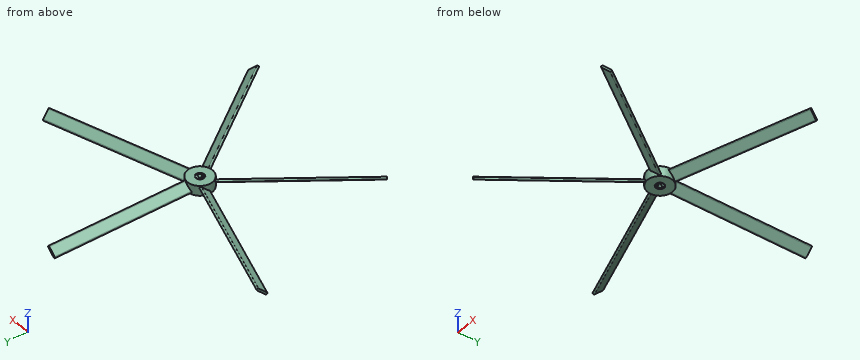
```python
from build123d import *

# Parameters (mm, degrees)
SKETCH1_R           = 7.5
SKETCH1_R_2         = 2.5
BOSS_EXTRUDE1_DEPTH = 6
BOSS_EXTRUDE2_DEPTH = 88.9
CIRPATTERN1_COUNT   = 5


with BuildPart() as part:
    # Sketch1 → Boss-Extrude1 (new body)
    with BuildSketch(Plane.XY):
        Circle(SKETCH1_R)
        Circle(SKETCH1_R_2, mode=Mode.SUBTRACT)
    extrude(amount=BOSS_EXTRUDE1_DEPTH)

    # Sketch3 → Boss-Extrude2 (add)
    with BuildSketch(Plane(origin=(0, 0, 0), x_dir=(1, 0, 0), z_dir=(0, 1, 0))):
        with BuildLine():
            Line((-2.427610564, -1.81062126), (1.710616437, -5.267397014))
            ThreePointArc((1.710616437, -5.267397014), (2.617021972, -5.186071015), (2.535695974, -4.27966548))
            Line((2.535695974, -4.27966548), (-1.602531027, -0.822889726))
            ThreePointArc((-1.602531027, -0.822889726), (-2.508936562, -0.904215725), (-2.427610564, -1.81062126))
        make_face()
    boss_extrude2 = extrude(amount=BOSS_EXTRUDE2_DEPTH)

    # CirPattern1: Boss-Extrude2 ×5 about axis
    cirpattern1_axis = Axis((0, 0, 0), (0, 0, 1))
    for i in range(1, CIRPATTERN1_COUNT):
        add(boss_extrude2.rotate(cirpattern1_axis, i * 360 / CIRPATTERN1_COUNT))


solid = part.part
```
Input: part model. Units: mm. Frame: model coordinates. Round coordinates to 2 decimals unless told otherwise and drop trailing zeros. Loops run counter-clockwise (first coordinate to the right, second up) from the corner with the lowest first, then second, coordinate; pieces in that order, holes last.
1) Pin query (flat end, axial travel): pin 1 (1.2 mm diameter, centred on x = -1, z = 1.5, fed in from -Y); pin 2 (1.5 mm diameter, centred on y = 54.5, z = 4, fed in from -X); pin 3 (4.5 mm diameter, centred on x = 0, y = 0, fed in from -Z); pin 4 (8 mm diameter, centred on x = 0, y = 0, fed in from -Z). Return the tip coordinate at first contact, or that it passes through.
Ans:
pin 1: stops at y = -7.49
pin 2: stops at x = -0.7
pin 3: stops at z = 0.67
pin 4: stops at z = 0
2) Section query A-A on y = 74. Return the cut outline in (x, z).
Ans:
outline: (-2.43, 1.81) arc R0.64 ccw to (-1.6, 0.82) - (2.54, 4.28) arc R0.64 ccw to (1.71, 5.27) - close
3) Material intervals for line 1 (Y direction, x = 0, z = 5.05) (1 decimal); line 2 (Y direction, x = 0, z = 5.25); line 3 (X direction, y = 33, z = 1.5), sorted ascending.
Ans:
line 1: y = -7.5 to -2.5, 1.5 to 7.5
line 2: y = -7.5 to -2.5, 1.78 to 7.5
line 3: x = -2.63 to -0.79
